Input: dimensioned drawing with shaded views. Units: mm. Origin: part minimum x, y, z. A direction names the side the tool comes from. Coordinates: 2 decimals unless noted, no trailing zeros. Order: outer loops, then holes, each group sorted by start corner. A loop starts at its lowest first (then second) coordinate and runs counter-clockwise, first axis right, second up. Notation, with made-up numbers: (-17.75, -10.75) - (37.25, -10.75) arc R17 cw to (37.25, 11.25) - close; hole circle Ø7 at (60.25, -1). An arc over 180 degrees is marked (long way). Use one line per item in the form item = value. Start each with the question number.
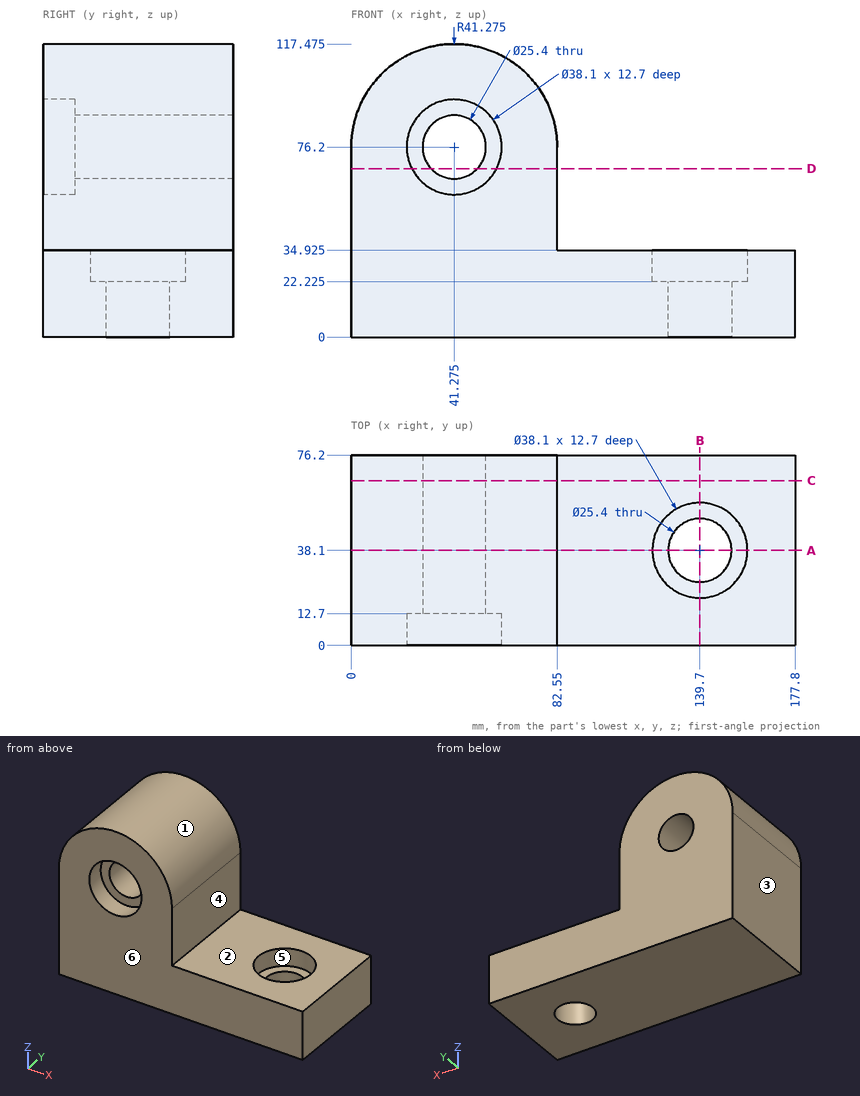
(1) Cut plane C-C on y = 66. Return the cut outline in (x, z) (3 decimals), plus the area to 3 significant figures.
(2) Cut plane D-D on z = 67.5. Return the cut outline in (x, y).
(3) Material intervals for L1, parallel to X at y = 38, z = 32; L2, parallel to X at y = 57, z = 76; L3, parallel to Y at x = 139, z = 16, sorted ascending. Write a range as from..to.
(4) Set-up query: the marked faces 1 and 2. Return all of +Z, -Z, +X, -X, +Y, -Y with unobstructed straight access to the full face (end or side cutting, diameter ignored); none if empty.
(5) Contact query for flat-ended pins moving along their axis: pin 1 Ø15 at (x, z) = (41.275, 76.2) entering from +Y; pin 2 Ø12.5 at (y, z) = (45, 57) entering from +X; pin 3 Ø10 at (x, z) = (53.5, 83) entering from -Y; pin 4 Ø10 at (x, y) = (82.5, 26) entering from +Z. Output: stop coordinate, or through.
(6) Cut plane A-A on y = 38.1. Return the cut outline in (x, z) (3 decimals), plus the area to 3 significant figures.
(7) Draft query along X for the marked faces 3, 4, 5 and 6. Return one class per face: released by +X, released by -X, zero draft, split by the parting line, or undercut.
(8) Cut plane B-B on x = 139.7. Return the cut outline in (y, z) (3 decimals).
Check sheet entries:
q1.outline = (0, 0) - (177.8, 0) - (177.8, 34.925) - (82.55, 34.925) - (82.55, 76.2) arc R41.275 ccw to (0, 76.2) - close; hole circle Ø25.4 at (41.275, 76.2)
q1.area = 11,800 mm^2
q2.outline = (0, 0) - (24.33, 0) - (24.33, 12.7) - (32.02, 12.7) - (32.02, 76.2) - (0, 76.2) - close; (50.53, 12.7) - (58.22, 12.7) - (58.22, 0) - (82.55, 0) - (82.55, 76.2) - (50.53, 76.2) - close
q3.L1 = 0..120.65, 158.75..177.8
q3.L2 = 0..28.58, 53.97..82.55
q3.L3 = 0..25.42, 50.78..76.2
q4.face_1 = +Z, +Y, -Y
q4.face_2 = +Z, +X, +Y, -Y
q5.pin_1 = through
q5.pin_2 = 82.55
q5.pin_3 = 12.7
q5.pin_4 = 95.98
q6.outline = (0, 0) - (127, 0) - (127, 22.225) - (120.65, 22.225) - (120.65, 34.925) - (82.55, 34.925) - (82.55, 76.2) arc R41.275 ccw to (0, 76.2) - close; (152.4, 0) - (177.8, 0) - (177.8, 34.925) - (158.75, 34.925) - (158.75, 22.225) - (152.4, 22.225) - close; hole circle Ø25.4 at (41.275, 76.2)
q6.area = 10,700 mm^2
q7.face_3 = released by -X
q7.face_4 = released by +X
q7.face_5 = undercut
q7.face_6 = zero draft
q8.outline = (0, 0) - (25.4, 0) - (25.4, 22.225) - (19.05, 22.225) - (19.05, 34.925) - (0, 34.925) - close; (50.8, 0) - (76.2, 0) - (76.2, 34.925) - (57.15, 34.925) - (57.15, 22.225) - (50.8, 22.225) - close
